The listing builds one solid part. Answer for the finished solid, in the listing's coordinates (mm). Face numbers are marked on the shaded views. A direction names the side the tool comes from. Give positions to 0.01 mm unless a question says otherwise; leave off trailing zeros. Write each loop counter-clockwise with the first axis right and the second up, starting at its lowest first coordinate (ties: lowest second). Pieces come first, ordered by that corner, then holes. Notation, with made-up numbers: M 65.5,31.25 L 74.5,31.25 A29 cw 74.5,52.25 Z; hole C -6,77 d8. An arc over 180 degrees is marked long. Return JSON: item names as keys, results as strings.
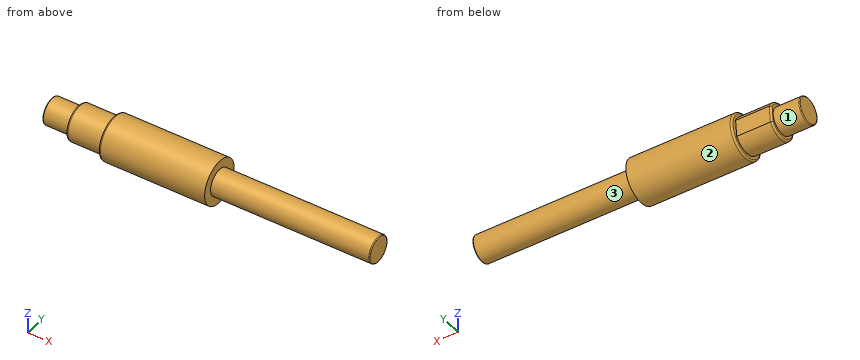
from build123d import *

# Parameters (mm, degrees)
SKETCH_1_R      = 1.5
EXTRUDE_1_DEPTH = 37
EXTRUDE_START   = -7
SKETCH_2_R      = 2.5
SKETCH_2_R_2    = 1
EXTRUDE_2_DEPTH = 12
EXTRUDE_START_2 = 3
SKETCH_3_R      = 1
EXTRUDE_4_DEPTH = 4
FILLET_1_R      = 0.1
FILLET_2_R      = 0.2


with BuildPart() as part:
    # 草图1 → 凸台-拉伸1 (new body)
    with BuildSketch(Plane(origin=(0, 0, 0), x_dir=(0, 0, -1), z_dir=(1, 0, 0))):
        Circle(SKETCH_1_R)
    extrude(amount=EXTRUDE_1_DEPTH)

    # 草图2 → 凸台-拉伸2 (add)
    with BuildSketch(Plane.ZY.offset(EXTRUDE_START)):
        Circle(SKETCH_2_R)
        Circle(SKETCH_2_R_2, mode=Mode.SUBTRACT)
    extrude(amount=-EXTRUDE_2_DEPTH)

    # 草图3 → 凸台-拉伸4 (add)
    with BuildSketch(Plane(origin=(0, 0, 0), x_dir=(0, 0, -1), z_dir=(1, 0, 0)).offset(EXTRUDE_START_2)):
        with BuildLine():
            Line((1.093724045, 1.674445494), (-0.720042675, 1.865888139))
            ThreePointArc((-0.720042675, 1.865888139), (-0.209933354, -1.988951479), (1.093724045, 1.674445494))
        make_face()
        Circle(SKETCH_3_R, mode=Mode.SUBTRACT)
    extrude(amount=EXTRUDE_4_DEPTH)

    # 圆角1
    fillet_1_edges = [part.edges().sort_by_distance(p)[0] for p in [
        (0, 0, 1.5),
        (37, 0, 1.5),
    ]]
    fillet(fillet_1_edges, radius=FILLET_1_R)

    # 圆角2
    fillet_2_edges = [part.edges().sort_by_distance(p)[0] for p in [
        (3, -1.988951479, 0.209933354),
        (3, 1.770166817, -0.186840685),
        (7, 0, -2.5),
    ]]
    fillet(fillet_2_edges, radius=FILLET_2_R)


solid = part.part
Item 1: Given pin 1 Ø1.5 at (x, z) = (17.5, -1.5) entering from +Y; pin 2 Ø1.5 at (x, y) = (10.5, 1) entering from -Z; pin 3 Ø1.5 at (x, y) = (20, 1.5) entering from -Z, each flat-ended and moving along its own axis, determine where each tip first touches the part or whether it passes through.
Geometry results:
{"pin 1": "stops at y = 2.38", "pin 2": "stops at z = -2.49", "pin 3": "stops at z = -1.3"}
Item 2: A cutting plane is placed at A-A, the plane x = 25. Write down the section's boundary in (y, z), plus the area to 3 significant figures.
Geometry results:
{"outline": "C 0,0 d3", "area": "7.07 mm2"}
Item 3: Which of the six approach directions +Z, -Z, +X, -X, +Y, -Y give full straight-line access (tool end or side, diameter ignored) to the marked faces 1, 2 and 3?
Geometry results:
{"face 1": "-X", "face 2": "+X, -X", "face 3": "+X"}
Item 4: Find the intervals of material crossed by line 1 (Y direction, x = 13, z = 1.5); line 2 (Y direction, x = 32, z = 0.1); line 3 (X direction, y = 0.85, z = 1.4), in increasing order.
Geometry results:
{"line 1": "y = -2 to 2", "line 2": "y = -1.5 to 1.5", "line 3": "x = 3 to 19"}
